```python
from build123d import *

# Parameters (mm, degrees)
SKETCH1_W           = 50.3
SKETCH1_H           = 50.3
BOSS_EXTRUDE1_DEPTH = 19
BOSS_EXTRUDE2_DEPTH = 5.55
BOSS_EXTRUDE3_DEPTH = 5.55
SKETCH5_R           = 3.175
BOSS_EXTRUDE4_DEPTH = 5.55
SKETCH7_R           = 2.75
BOSS_EXTRUDE5_DEPTH = 5.55
SKETCH8_R           = 1.59
CUT_EXTRUDE1_DEPTH  = 20


with BuildPart() as part:
    # Sketch1 → Boss-Extrude1 (new body)
    with BuildSketch(Plane(origin=(0, 0, 0), x_dir=(1, 0, 0), z_dir=(0, 1, 0))):
        Rectangle(SKETCH1_W, SKETCH1_H)
    extrude(amount=BOSS_EXTRUDE1_DEPTH)

    # Sketch2 → Boss-Extrude2 (add)
    with BuildSketch(Plane.XY.offset(25.15)):
        Polygon((-15.692878403, 14.649004006), (-18.635756806, 9.551789092), (-15.692878403, 4.454574178), (-9.807121597, 4.454574178), (-6.864243194, 9.551789092), (-9.807121597, 14.649004006), align=None)
        Polygon((18.635756806, 9.551789092), (15.692878403, 4.454574178), (9.807121597, 4.454574178), (6.864243194, 9.551789092), (9.807121597, 14.649004006), (15.692878403, 14.649004006), align=None)
    extrude(amount=BOSS_EXTRUDE2_DEPTH)

    # Sketch4 → Boss-Extrude3 (add)
    with BuildSketch(Plane(origin=(0, 0, -25.15), x_dir=(-1, 0, 0), z_dir=(0, 0, -1))):
        Polygon((-5.835508644, 9.984378867), (-2.892754322, 4.887378867), (2.992754322, 4.887378867), (5.935508644, 9.984378867), (2.992754322, 15.081378867), (-2.892754322, 15.081378867), align=None)
    extrude(amount=BOSS_EXTRUDE3_DEPTH)

    # Sketch5 → Boss-Extrude4 (add)
    with BuildSketch(Plane(origin=(0, 0, -30.7), x_dir=(-1, 0, 0), z_dir=(0, 0, -1))):
        with Locations((0, 9.996378867)):
            Circle(SKETCH5_R)
    extrude(amount=BOSS_EXTRUDE4_DEPTH)

    # Sketch7 → Boss-Extrude5 (add)
    with BuildSketch(Plane.XY.offset(30.7)):
        with Locations((-12.750756806, 9.564004006)):
            Circle(SKETCH7_R)
        with Locations((12.750756806, 9.564004006)):
            Circle(SKETCH7_R)
    extrude(amount=BOSS_EXTRUDE5_DEPTH)

    # Sketch8 → Cut-Extrude1 (cut, through all)
    with BuildSketch(Plane(origin=(0, 19, 0), x_dir=(1, 0, 0), z_dir=(0, 1, 0))):
        with Locations((-22.25, 0)):
            Circle(SKETCH8_R)
        with Locations((22.25, 0)):
            Circle(SKETCH8_R)
    extrude(amount=-CUT_EXTRUDE1_DEPTH, mode=Mode.SUBTRACT)


solid = part.part
```
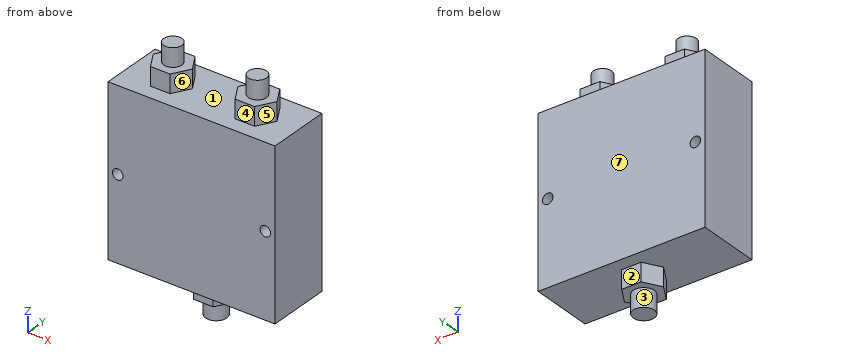
Geometry: final body of the model. Coordinates: model frame, mm. Face numbers are marked on the shaded views. A direction names the side the tool comes from. Round coordinates to 2 decimals unless told otherwise and drop trailing zeros. Loops run counter-clockwise (first coordinate to the right, second up) from the corner with the lowest first, then second, coordinate; pieces in that order, holes last.
Item 1: Section C-C, the plane x = 0. Output: boundary loops of the cut face in (y, z), plus the area to 3 significant figures.
Checked values:
outline: (0, -25.15) - (4.89, -25.15) - (4.89, -30.7) - (6.82, -30.7) - (6.82, -36.25) - (13.17, -36.25) - (13.17, -30.7) - (15.08, -30.7) - (15.08, -25.15) - (19, -25.15) - (19, 25.15) - (0, 25.15) - close
area: 1,050 mm2
Item 2: Mould query, pull axis X, two halves, no side actions, for the marked faces 5, 6 and 7. Classes: released by +X, released by -X, zero draft, split by the parting line, or undercut.
Checked values:
face 5: released by +X
face 6: undercut
face 7: zero draft
Item 3: Contact query for flat-ended pins moving along their axis: P1, Ø5, axis at x = 8.5, y = 9.5, coming from the -Z side; P2, Ø3, axis at x = -22.25, z = 0, coming from the +Y side; P3, Ø1.7, axis at x = -14, z = 28.5, coming from the -Y side; P4, Ø3, axis at x = -13.5, z = 27.5, coming from the +Y side. Output: stop coordinate, or through.
Checked values:
P1: stops at z = -25.15
P2: passes through
P3: stops at y = 4.45
P4: stops at y = 14.65
Item 4: Section A-A, the plane x = 22.25. Output: boundary loops of the cut face in (y, z), plus the area to 3 significant figures.
Checked values:
outline: (0, -25.15) - (19, -25.15) - (19, -1.59) - (0, -1.59) - close; (0, 1.59) - (19, 1.59) - (19, 25.15) - (0, 25.15) - close
area: 895 mm2
Item 5: Section D-D, the plane y = 2. Output: boundary loops of the cut face in (x, z).
Checked values:
outline: (-25.15, -25.15) - (25.15, -25.15) - (25.15, 25.15) - (-25.15, 25.15) - close; hole circle Ø3.18 at (-22.25, 0); hole circle Ø3.18 at (22.25, 0)
Item 6: Reachability of the marked faces 1, 2, 3 and 4 from +Z, -Z, +X, -X, +Y, -Y: full face, straight path, thin tool, end or side. Return the list, or none.
Checked values:
face 1: +Z
face 2: -Z, +X, -X, +Y
face 3: -Z
face 4: +Z, +X, -X, -Y
Item 7: Line query: L1, parallel to X at y = 13.25, z = 0; L2, parallel to Z at x = 22.25, y = 9; L3, parallel to Z at x = 19.5, y = 14.25. Output: solid intervals per line, ascending.
Checked values:
L1: x = -25.15 to -23.84, -20.66 to 20.66, 23.84 to 25.15
L2: z = -25.15 to -1.59, 1.59 to 25.15
L3: z = -25.15 to 25.15
Item 8: Section B-B, the plane z = 26.5. Output: boundary loops of the cut face in (x, y).
Checked values:
outline: (-18.64, 9.55) - (-15.69, 4.45) - (-9.81, 4.45) - (-6.86, 9.55) - (-9.81, 14.65) - (-15.69, 14.65) - close; (6.86, 9.55) - (9.81, 4.45) - (15.69, 4.45) - (18.64, 9.55) - (15.69, 14.65) - (9.81, 14.65) - close
